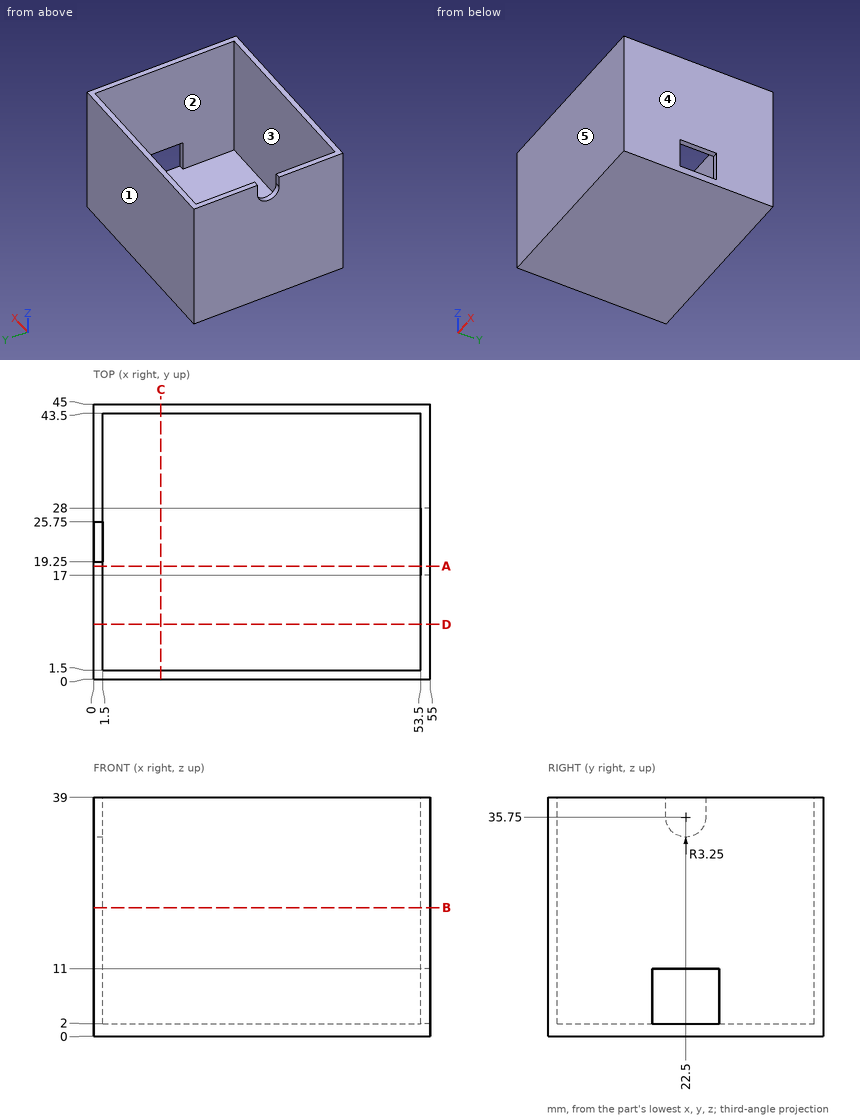
Answer from the drawing. Dimensions are ordinates in mm from the lowest x, y and z of the part. A direction names the side the tool comes from. Coordinates: 2 decimals unless noted, no trailing zeros. Write each loop counter-clockwise with the first axis right and the second up, starting at its lowest first coordinate (ties: lowest second). Pieces come first, ordered by that corner, then holes. Notation, with made-up numbers: M -10.5,-27 L 36.5,-27 A14 ccw 36.5,-1 Z; hole C 33,-7.75 d11. An arc over 180 degrees is marked long. Use a Markdown table: item, result.
Q1. The part is cut by section C-C, the plane x = 11. Write down the section's boundary in (y, z).
Answer block:
| item | result |
|---|---|
| outline | M 0,0 L 45,0 L 45,39 L 43.5,39 L 43.5,2 L 1.5,2 L 1.5,39 L 0,39 Z |
Q2. Which of the six approach directions +Z, -Z, +X, -X, +Y, -Y give full straight-line access (tool end or side, diameter ignored) to the marked faces 1 and 2?
Answer block:
| item | result |
|---|---|
| face 1 | +Z, -Z, +X, -X, +Y |
| face 2 | +Z |
Q3. The part is cut by section B-B, the plane z = 21. Write down the section's boundary in (x, y), then the cut area to 3 significant figures.
Answer block:
| item | result |
|---|---|
| outline | M 0,0 L 55,0 L 55,45 L 0,45 Z; hole M 1.5,1.5 L 53.5,1.5 L 53.5,43.5 L 1.5,43.5 Z |
| area | 291 mm2 |
Q4. The part is cut by section D-D, the plane y = 9. Write down the section's boundary in (x, z).
Answer block:
| item | result |
|---|---|
| outline | M 0,0 L 55,0 L 55,39 L 53.5,39 L 53.5,2 L 1.5,2 L 1.5,39 L 0,39 Z |
Q5. Straight lines are drawn through the part: L1, parallel to Y at x = 11.5, z = 31; L2, parallel to X at y = 40, z = 36; L3, parallel to X at y = 25.5, z = 8.5. For each, find the intervals that lie inside material, in ascending order. Write a range as [from, to].
Answer block:
| item | result |
|---|---|
| L1 | y = [0, 1.5], [43.5, 45] |
| L2 | x = [0, 1.5], [53.5, 55] |
| L3 | x = [0, 1.5] |
Q6. Determine the mould class of the marked faces 3, 4 and 5 for opening direction Y: released by +Y, released by -Y, zero draft, split by the parting line, or undercut.
Answer block:
| item | result |
|---|---|
| face 3 | undercut |
| face 4 | zero draft |
| face 5 | released by -Y |
Q7. The part is cut by section A-A, the plane y = 18.5. Write down the section's boundary in (x, z).
Answer block:
| item | result |
|---|---|
| outline | M 0,0 L 55,0 L 55,2 L 1.5,2 L 1.5,39 L 0,39 Z; M 53.5,11 L 55,11 L 55,39 L 53.5,39 Z |
Q8. This flat-tipped pin is pushed along its axis until it touches: pin 1 Ø1 at (x, y) = (19.5, 14) entering from +Z. Where does it stop, or does it pass through?
Answer block:
| item | result |
|---|---|
| pin 1 | stops at z = 2 |
